from build123d import *

# Parameters (mm, degrees)
PAD_DEPTH       = 6
SKETCH001_W     = 140.7
SKETCH001_H     = 1.6
POCKET_DEPTH    = 4.5
SKETCH002_R     = 1.5
POCKET001_DEPTH = 4.001


with BuildPart() as part:
    # Sketch → Pad (new body)
    with BuildSketch(Plane.XY):
        Polygon((-71.25, 2), (-71.25, -2), (-66.75, -2), (-66.25, -1.5), (-5, -1.5), (-4.5, -2), (4.5, -2), (5, -1.5), (66.25, -1.5), (66.75, -2), (71.25, -2), (71.25, 2), (66.75, 2), (66.25, 1.5), (5, 1.5), (4.5, 2), (-4.5, 2), (-5, 1.5), (-66.25, 1.5), (-66.75, 2), align=None)
    extrude(amount=PAD_DEPTH)

    # Sketch001 (on Face22 of Pad) → Pocket (cut)
    with BuildSketch(Plane.XY.offset(6)):
        Rectangle(SKETCH001_W, SKETCH001_H)
    extrude(amount=-POCKET_DEPTH, mode=Mode.SUBTRACT)

    # Sketch002 (on Face10 of Pocket) → Pocket001 (cut, through all)
    with BuildSketch(Plane.XZ.offset(2)):
        with Locations((-68.625, 3.65)):
            Circle(SKETCH002_R)
        with Locations((-2.625, 3.65)):
            Circle(SKETCH002_R)
        with Locations((2.625, 3.65)):
            Circle(SKETCH002_R)
        with Locations((68.625, 3.65)):
            Circle(SKETCH002_R)
        Polygon((-66.75, 6), (-66.25, 3.5), (-5, 3.5), (-4.5, 6), align=None)
        Polygon((4.5, 6), (5, 3.5), (66.25, 3.5), (66.75, 6), align=None)
    extrude(amount=-POCKET001_DEPTH, mode=Mode.SUBTRACT)


solid = part.part
Geometry: final body of the model. Coordinates: model frame, mm. A direction names the side the tool comes from. Coordinates: 2 decimals unless noted, no trailing zeros. Order: outer loops, then holes, each group sorted by start corner. A loop starts at its lowest first (then second) coordinate and runs counter-clockwise, first axis right, second up.
1) Section A-A (x = -9). Return loops of the section in (y, z).
Result sheet:
outline: (-1.5, 0) - (1.5, 0) - (1.5, 3.5) - (0.8, 3.5) - (0.8, 1.5) - (-0.8, 1.5) - (-0.8, 3.5) - (-1.5, 3.5) - close
2) Draft query along Z for faces 6 (the cylindrical face through (-1.239, 1.392, 3.075)), 7 (the flat face through (69, -2, 2)), 8 (the flat face through (-69, 1, 6)). Return one class per face: released by +Z, released by -Z, zero draft, split by the parting line, or undercut.
Result sheet:
face 6: undercut
face 7: zero draft
face 8: released by +Z
3) Set-up query: faces 1 (the cylindrical face through (70.056, 1.392, 4.101)), 2 (the flat face through (35, -1.5, 2)), 3 (the flat face through (69, 1, 6)), 4 (the flat face through (-1, 0.8, 3)), 5 (the flat face through (-35, 1.5, 2)). Return all of +Z, -Z, +X, -X, +Y, -Y with unobstructed straight access to the full face (end or side cutting, diameter ignored); none if empty.
Result sheet:
face 1: +Y, -Y
face 2: +Z, -Z, -Y
face 3: +Z, +X, -X, +Y, -Y
face 4: +Z
face 5: +Z, -Z, +Y
4) Ray query, probe 1 along X at (y, z) = (1.45, 2.5); probe 2 along Y at (x, z) = (62, 3.25); probe 3 along Y at (x, z) = (-1, 2.5). Return the intervals inside material, ascending.
Result sheet:
probe 1: x = -71.25 to -69.59, -67.66 to -3.59, -1.66 to 1.66, 3.59 to 67.66, 69.59 to 71.25
probe 2: y = -1.5 to -0.8, 0.8 to 1.5
probe 3: y = -2 to -0.8, 0.8 to 2
5) First-contact query: P1, Ø1, axis at x = 25, y = 0, coming from the +Z side; P2, Ø3, axis at x = -24, z = 2, coming from the +Y side; P3, Ø1, axis at x = -18.5, y = -1.5, coming from the +Z side; P4, Ø1.5, axis at x = -35, y = 0, coming from the -Z side. Flat tips, straight axial feed; report the tip coordinate or a pass-through.
Result sheet:
P1: stops at z = 1.5
P2: stops at y = 1.5
P3: stops at z = 3.5
P4: stops at z = 0
